Autodesk Inventor part; units mm, degrees
ref_plane "YZ Plane" through (0, 0, 0) normal (1, 0, 0) x (0, 1, 0)
ref_plane "XZ Plane" through (0, 0, 0) normal (0, 1, 0) x (-1, 0, 0)
ref_plane "XY Plane" through (0, 0, 0) normal (0, 0, 1) x (1, 0, 0)
sketch "Sketch1" plane through (0, 0, 0) normal (0, 0, 1) x (1, 0, 0)
  circle A0 centre (0, 0) radius 12.7
  dimension "d0" = 25.4
extrude "Extrusion1" add sketch "Sketch1" along normal blind 380
sketch "Sketch2" plane through (0, 0, 0) normal (0, 0, -1) x (-1, 0, 0)
  circle A0 centre (0, 0) radius 12.7 construction
  circle A1 centre (0, 0) radius 4
  dimension "d3" = 8
extrude "Extrusion2" add sketch "Sketch2" along normal blind 20
thread "Thread1"
chamfer "Chamfer1" distance 2 angle 45 1 edges at (-12.7, 0, 380)
properties part number "22-130 RAIL" material "Aluminum-6061"
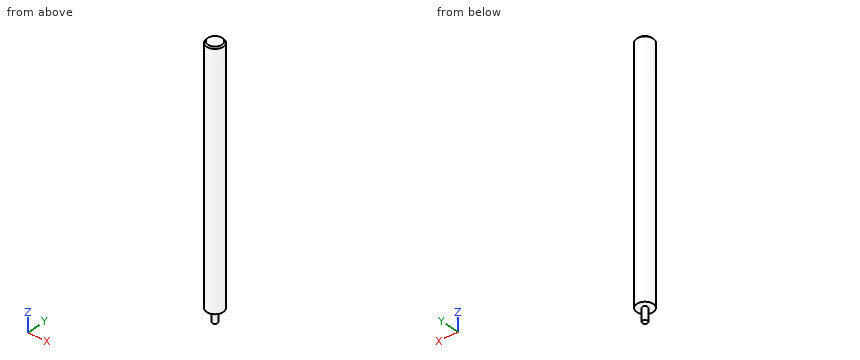
For this review, take the finished solid that the model builds, in its own axes (mm). Give positions to 0.01 mm unless a question says otherwise; leave off trailing zeros. Loops run counter-clockwise (first coordinate to the right, second up) from the corner with the lowest first, then second, coordinate; pieces in that order, holes last. Notation, with made-up numbers: M 21,49.5 L 73,49.5 A12 ccw 73,71.5 Z; hole C 65.5,51 d4. An arc over 180 degrees is marked long. Answer as a JSON object with one key per item and string values. Group by question number.
Q1. For probe 1 along Z at (x, y) = (7.5, -2.75); probe 2 along Y at (x, z) = (-0.25, 163); probe 3 along X at (y, z) = (9.25, 105), list the stretches that pass through material, from the lowest coordinate up. Write a range as [from, to].
Q2. Add section C-C on z = 43. Give the boundary of the cut face in (x, y), and give its area (3 significant figures).
Q3. Insertion check: P1, Ø1.5, axis at x = 5, z = 57.5, coming from the +Y side; P2, Ø1, axis at x = -2.5, z = 58, coming from the -Y side; P3, Ø6, axis at x = -3, y = -9, coming from the -Z side; P4, Ø10, axis at y = -3.5, z = 33.5, coming from the -X side. Each pin has a flat end and moves straight along its axis. Give the tip position at first contact, or say it passes through.
Q4. Add section A-A on x = 0. Give the boundary of the cut face in (y, z), and give its area (3 significant figures).
Checked values:
{
 "1": {"probe 1": "[0, 380]", "probe 2": "[-12.7, 12.7]", "probe 3": "[-8.7, 8.7]"},
 "2": {"outline": "C 0,0 d25.4", "area": "507 mm²"},
 "3": {"P1": "y = 11.97", "P2": "y = -12.54", "P3": "z = 0", "P4": "x = -12.7"},
 "4": {"outline": "M -12.7,0 L -4,0 L -4,-20 L 4,-20 L 4,0 L 12.7,0 L 12.7,378 L 10.7,380 L -10.7,380 L -12.7,378 Z", "area": "9,810 mm²"}
}
